Geometry: final body of the model. Coordinates: model frame, mm. A direction names the side the tool comes from. Give positions to 0.01 mm unless a question says otherwise; leave off trailing zeros. Write each loop counter-clockwise with the first axis right and the second up, starting at its lowest first coordinate (ties: lowest second). Pieces come first, ordered by that corner, then holes.
Q1. Section D-D (x = -35.5). Return the cut outline in (y, z).
Q2. Mould query, pull axis Y, two halves, no side actions, for faces 1 (the cylindrical face through (11.604, 23.851, -1.972)), 2 (the flat face through (-23, 10, -4)), 3 (the flat face through (16.423, 16.794, -1.972)). Classes: +Y half, -Y half, draft (parallel to the pull), parting line (faces both ways), or undercut.
Q3. Section A-A (x = 0). Return the cut outline in (y, z), plus the area to 3 significant figures.
Q4. Line query: line 1 (Y direction, x = 0, z = -1.3); line 2 (X direction, y = 4.5, z = -0.5); line 3 (X direction, y = -2, z = -1.65). Output: solid intervals per line, ascending.
Q5. Section C-C (z = -1.1). Return the cut outline in (x, y), plus the area to 3 significant figures.
Q6. Pin query (flat end, axial travel): pin 1 Ø1.5 at (y, z) = (-14, -0.5) entering from -X. Return the tip coordinate at first contact, or that it passes through.
Q7. Reachability of faces 4 (the flat face through (-43, 29.5, -2)), 5 (the cylindrical face through (-49.124, -16.606, -1.972)) from +Z, -Z, +X, -X, +Y, -Y: full face, straight path, thin tool, end or side. Return the list, or none.
Q8. Section B-B (y = 25). Return the cut outline in (x, z).
from build123d import *

# Parameters (mm, degrees)
SKETCH_1_R             = 6
SKETCH_1_R_2           = 3
SM_BASE_FLANGE_1_DEPTH = 4


# Sheet-metal steps are written as plain solids
with BuildPart() as part:
    # Sketch 1 → Базовая кромка1 (new body)
    with BuildSketch(Plane.XY):
        with BuildLine():
            Line((-94.18015229, 29.5), (0, 29.5))
            Line((0, 29.5), (8.832749987, 29.5))
            ThreePointArc((8.832749987, 29.5), (11.445095498, 28.664103019), (13.086929131, 26.466955969))
            Line((13.086929131, 26.466955969), (19.852836003, 6.845794522))
            ThreePointArc((19.852836003, 6.845794522), (3.470622706, -20.71122348), (-21, 0))
            ThreePointArc((-21, 0), (-35.5, 14.5), (-50, 0))
            ThreePointArc((-50, 0), (-49.640340933, -5.986363846), (-48.566537916, -11.88660569))
            ThreePointArc((-48.566537916, -11.88660569), (-49.156122287, -16.666789945), (-52.76892738, -19.85197606))
            Line((-52.76892738, -19.85197606), (-94.18015229, 29.5))
        make_face()
        Circle(SKETCH_1_R, mode=Mode.SUBTRACT)
        with Locations((8.832749987, 25)):
            Circle(SKETCH_1_R_2, mode=Mode.SUBTRACT)
    extrude(amount=-SM_BASE_FLANGE_1_DEPTH)


solid = part.part
Computed:
1. outline: (14.5, -4) - (29.5, -4) - (29.5, 0) - (14.5, 0) - close
2. face 1: undercut
2. face 2: draft
2. face 3: +Y half
3. outline: (-21, -4) - (-6, -4) - (-6, 0) - (-21, 0) - close; (6, -4) - (29.5, -4) - (29.5, 0) - (6, 0) - close
3. area: 154 mm2
4. line 1: y = -21 to -6, 6 to 29.5
4. line 2: x = -73.2 to -49.28, -21.72 to -3.97, 3.97 to 20.51
4. line 3: x = -67.75 to -49.96, -20.9 to -5.66, 5.66 to 20.9
5. outline: (-94.18, 29.5) - (-52.77, -19.85) arc R6.79 ccw to (-48.57, -11.89) arc R50 cw to (-50, 0) arc R14.5 cw to (-21, 0) arc R21 ccw (long way) to (19.85, 6.85) - (13.09, 26.47) arc R4.5 ccw to (8.83, 29.5) - close; hole circle Ø12 at (0, 0); hole circle Ø6 at (8.83, 25)
5. area: 3,370 mm2
6. pin 1: stops at x = -58.31
7. face 4: +Z, -Z, +X, -X, +Y
7. face 5: +Z, -Z
8. outline: (-90.4, -4) - (5.83, -4) - (5.83, 0) - (-90.4, 0) - close; (11.83, -4) - (13.59, -4) - (13.59, 0) - (11.83, 0) - close
